```python
from build123d import *

# Parameters (mm, degrees)
SKETCH1_R           = 6.5
BOSS_EXTRUDE1_DEPTH = 1.5
SKETCH2_R           = 5.8
BOSS_EXTRUDE2_DEPTH = 9
FILLET1_R           = 0.4
SKETCH3_R           = 5
CUT_EXTRUDE1_DEPTH  = 4.8
BOSS_EXTRUDE3_DEPTH = 4.8
SKETCH5_W           = 2
SKETCH5_H           = 0.8
SKETCH5_W_2         = 1
SKETCH5_H_2         = 3.8
BOSS_EXTRUDE4_DEPTH = 7.2
CUT_EXTRUDE2_REACH  = 10.4
BOSS_EXTRUDE5_DEPTH = 3.8
FILLET2_R           = 0.1
FILLET3_R           = 0.2


with BuildPart() as part:
    # Sketch1 → Boss-Extrude1 (new body)
    with BuildSketch(Plane(origin=(0, 0, 0), x_dir=(1, 0, 0), z_dir=(0, 1, 0))):
        Circle(SKETCH1_R)
    extrude(amount=BOSS_EXTRUDE1_DEPTH)

    # Sketch2 → Boss-Extrude2 (add)
    with BuildSketch(Plane(origin=(0, 1.5, 0), x_dir=(1, 0, 0), z_dir=(0, 1, 0))):
        Circle(SKETCH2_R)
    extrude(amount=BOSS_EXTRUDE2_DEPTH)

    # Fillet1
    fillet1_edges = [part.edges().sort_by_distance(p)[0] for p in [
        (-5.8, 10.5, 0),
    ]]
    fillet(fillet1_edges, radius=FILLET1_R)

    # Sketch3 → Cut-Extrude1 (cut)
    with BuildSketch(Plane.XZ):
        Circle(SKETCH3_R)
    extrude(amount=-CUT_EXTRUDE1_DEPTH, mode=Mode.SUBTRACT)

    # Sketch4 → Boss-Extrude3 (add)
    with BuildSketch(Plane.XZ.offset(-4.8)):
        with BuildLine():
            Line((-4.990991885, 0.3), (-2.9, 0.3))
            Line((-2.9, 0.3), (-2.9, -0.3))
            Line((-2.9, -0.3), (-4.990991885, -0.3))
            ThreePointArc((-4.990991885, -0.3), (-5, 0), (-4.990991885, 0.3))
        make_face()
        with BuildLine():
            Line((2.9, 0.3), (2.9, -0.3))
            Line((2.9, -0.3), (4.990991885, -0.3))
            ThreePointArc((4.990991885, -0.3), (5, 0), (4.990991885, 0.3))
            Line((4.990991885, 0.3), (2.9, 0.3))
        make_face()
        with BuildLine():
            Line((-0.3, 4.990991885), (-0.3, 2.7))
            Line((-0.3, 2.7), (0.3, 2.7))
            Line((0.3, 2.7), (0.3, 4.990991885))
            ThreePointArc((0.3, 4.990991885), (0, 5), (-0.3, 4.990991885))
        make_face()
        with BuildLine():
            Line((0.3, -2.7), (-0.3, -2.7))
            Line((-0.3, -2.7), (-0.3, -4.990991885))
            ThreePointArc((-0.3, -4.990991885), (0, -5), (0.3, -4.990991885))
            Line((0.3, -4.990991885), (0.3, -2.7))
        make_face()
    extrude(amount=BOSS_EXTRUDE3_DEPTH)

    # Sketch5 → Boss-Extrude4 (add)
    with BuildSketch(Plane.XZ.offset(-4.8)):
        with Locations((0, 2.3)):
            Rectangle(SKETCH5_W, SKETCH5_H)
        with Locations((-2.4, 0)):
            Rectangle(SKETCH5_W_2, SKETCH5_H_2)
        with Locations((2.4, 0)):
            Rectangle(SKETCH5_W_2, SKETCH5_H_2)
        with Locations((0, -2.3)):
            Rectangle(SKETCH5_W, SKETCH5_H)
    extrude(amount=BOSS_EXTRUDE4_DEPTH)

    # Sketch6 → Cut-Extrude2 (cut, up to next)
    with BuildSketch(Plane.XY.offset(1.9), mode=Mode.PRIVATE) as cut_extrude2_sk1:
        Polygon((-1.9, -2.4), (-1.9, -1.9625), (-2.4, -2.4), align=None)
    cut_extrude2_tool1 = extrude(cut_extrude2_sk1.sketch, amount=-CUT_EXTRUDE2_REACH, mode=Mode.PRIVATE) & part.part
    add(cut_extrude2_tool1.solids().sort_by_distance((-2.066667, -2.254167, 1.9))[0], mode=Mode.SUBTRACT)
    # Sketch6 → Cut-Extrude2 (cut, up to next)
    with BuildSketch(Plane.XY.offset(1.9), mode=Mode.PRIVATE) as cut_extrude2_sk2:
        Polygon((1.9, -1.9625), (1.9, -2.4), (2.4, -2.4), align=None)
    cut_extrude2_tool2 = extrude(cut_extrude2_sk2.sketch, amount=-CUT_EXTRUDE2_REACH, mode=Mode.PRIVATE) & part.part
    add(cut_extrude2_tool2.solids().sort_by_distance((2.066667, -2.254167, 1.9))[0], mode=Mode.SUBTRACT)

    # Sketch6<3> → Boss-Extrude5 (add)
    with BuildSketch(Plane.XY.offset(1.9)):
        Polygon((-1.6, -1.7), (-1.9, -1.4), (-1.9, -1.9625), align=None)
        Polygon((1.6, -1.7), (1.9, -1.9625), (1.9, -1.4), align=None)
    extrude(amount=-BOSS_EXTRUDE5_DEPTH)

    # Fillet2
    fillet2_edges = [part.edges().sort_by_distance(p)[0] for p in [
        (-1.6, -1.7, 0),
        (1.6, -1.7, 0),
    ]]
    fillet(fillet2_edges, radius=FILLET2_R)

    # Fillet3
    fillet3_edges = [part.edges().sort_by_distance(p)[0] for p in [
        (-6.5, 1.5, 0),
    ]]
    fillet(fillet3_edges, radius=FILLET3_R)


solid = part.part
```
Can you work these out from the model? Positions are in its coordinate system, mm. A direction names the side the tool comes from. Give positions to 0.01 mm unless a question says otherwise; leave off trailing zeros. Write each loop counter-clockwise with the first axis right and the second up, starting at its lowest first coordinate (ties: lowest second). Pieces come first, ordered by that corner, then holes. Notation, with made-up numbers: (-9.75, 24.25) -> (26.25, 24.25) arc R35 cw to (26.25, 63.25) -> close; hole circle Ø1 at (8.5, -20.75). An arc over 180 degrees is marked (long way). One line per item, written item: value.
Q1. Please list where these lines run through material, in increasing order: line 1 (X direction, y = -0.5, z = 1.5); line 2 (X direction, y = 2.5, z = -2.75); line 3 (Y direction, x = 1.25, z = -3.5). Write a range as [from, to].
Results found:
line 1: x = [-2.9, -1.9], [1.9, 2.9]
line 2: x = [-5.11, -4.18], [-0.3, 0.3], [4.18, 5.11]
line 3: y = [4.8, 10.5]
Q2. Imagine slicing it at C-C on x = 0. Please give me the cut outline in (y, z), and give its area (3 significant figures).
Results found:
outline: (-2.4, -2.7) -> (0, -2.7) -> (0, -6.5) -> (1.3, -6.5) arc R0.2 ccw to (1.5, -6.3) -> (1.5, -5.8) -> (10.1, -5.8) arc R0.4 ccw to (10.5, -5.4) -> (10.5, 5.4) arc R0.4 ccw to (10.1, 5.8) -> (1.5, 5.8) -> (1.5, 6.3) arc R0.2 ccw to (1.3, 6.5) -> (0, 6.5) -> (0, 2.7) -> (-2.4, 2.7) -> (-2.4, 1.9) -> (4.8, 1.9) -> (4.8, -1.9) -> (-2.4, -1.9) -> close
area: 109 mm^2
Q3. Which directions (+Z, -Z, +X, -X, +Y, -Y) give clear straight access to the entire face, cutting with the end or side of a thin tool? Please do faces 1 (the face through (-1.9, 2, 0)), 2 (the face through (-4, 2, -3)).
Results found:
face 1: none
face 2: -Y
Q4. We'd pull the mould along Z, two halves only. Please class faces 3 (the face through (4, 2, -0.3)), 4 (the face through (0, 0, -3)): +Z half, -Z half, draft (parallel to the pull), parting line (faces both ways), or undercut.
Results found:
face 3: undercut
face 4: draft
Q5. Imagine slicing it at B-B on z = 0. Please give me the cut outline in (x, y).
Results found:
outline: (-6.5, 0) -> (-2.9, 0) -> (-2.9, -2.4) -> (-2.4, -2.4) -> (-1.68, -1.77) arc R0.1 ccw to (-1.68, -1.62) -> (-1.9, -1.4) -> (-1.9, 4.8) -> (1.9, 4.8) -> (1.9, -1.4) -> (1.68, -1.62) arc R0.1 ccw to (1.68, -1.77) -> (2.4, -2.4) -> (2.9, -2.4) -> (2.9, 0) -> (6.5, 0) -> (6.5, 1.3) arc R0.2 ccw to (6.3, 1.5) -> (5.8, 1.5) -> (5.8, 10.1) arc R0.4 ccw to (5.4, 10.5) -> (-5.4, 10.5) arc R0.4 ccw to (-5.8, 10.1) -> (-5.8, 1.5) -> (-6.3, 1.5) arc R0.2 ccw to (-6.5, 1.3) -> close
Q6. For P1, Ø0.6, axis at x = 0, y = 2, coming from the -Z side; P2, Ø1.4, axis at x = 2, y = 1, coming from the +Z side; P3, Ø4, axis at y = -1, z = -3, coming from the -X side, each with a flat end and sliding along its axis, tell me the tip position at first contact or that it passes through.
Results found:
P1: stops at z = -5.8
P2: stops at z = 6.37
P3: stops at x = -6.38
